Can you work these out from the drawing? Everything is in mm from the part's minimum corner. A direction names the side the tool comes from. Round coordinates to 2 decimals unless told otherwise and drop trailing zeros. Order: outer loops, then holes, each group sorted by start corner. A loop starts at its lowest first (then second) coordinate and runs counter-clockwise, first axis right, second up. Notation, with made-up numbers: (28, -23) - (56, -23) arc R28 cw to (56, 3) - close; hole circle Ø2 at (58.5, -0.75). An arc over 180 degrees is marked (long way). Write item = value, one per line.
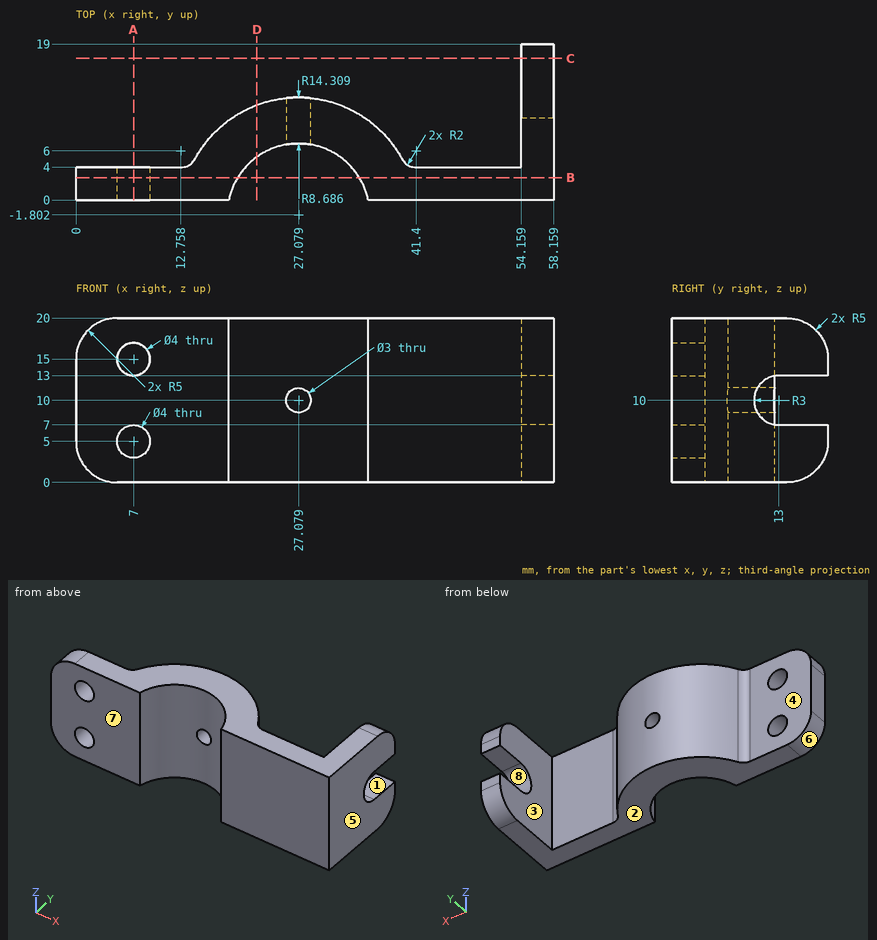
(1) On a 3-axis mill with a long thin cutter (end or side, diameter ignored), from which of +Z, -Z, +X, -X, +Y, -Y can I reach the whole of each face in a straight line? I mean the marked faces 1, 2, 3, 4 and 5. Say none if no direction works.
Computed:
face_1 = +X, -X, +Y
face_2 = -Z, +X, -X, +Y, -Y
face_3 = +Z, -Z, +Y
face_4 = +Z, -Z, -X, +Y
face_5 = +Z, -Z, +X, +Y, -Y
(2) Will these pins go through, and if not, where does the flat tip stop? P1, Ø3, axis at x = 56.5, y = 16, coming from the -Z side (1 decimal); P2, Ø10, axis at x = 6, z = 8, coming from the +Y side; P3, Ø3.5, axis at x = 7, z = 5, coming from the -Y side; P4, Ø5, axis at x = 7, z = 15, coming from the -Y side.
Computed:
P1 = 0
P2 = 4
P3 = through
P4 = 0
(3) If we section it at D-D (x = 22): Write out the boundary of the cut face in (y, z) (1 decimal).
Computed:
outline = (5.2, 0) - (11.6, 0) - (11.6, 20) - (5.2, 20) - close
(4) If we section it at B-B (y = 2.75): Write out the boundary of the cut face in (x, z).
Computed:
outline = (0, 5) arc R5 ccw to (5, 0) - (19.68, 0) - (19.68, 20) - (5, 20) arc R5 ccw to (0, 15) - close; (34.48, 0) - (58.16, 0) - (58.16, 20) - (34.48, 20) - close; hole circle Ø4 at (7, 5); hole circle Ø4 at (7, 15)
(5) If we section it at A-A (x = 7): Write out the boundary of the cut face in (y, z).
Computed:
outline = (0, 0) - (4, 0) - (4, 3) - (0, 3) - close; (0, 7) - (4, 7) - (4, 13) - (0, 13) - close; (0, 17) - (4, 17) - (4, 20) - (0, 20) - close
(6) Thinking about a two-plate mould opening in Z: for the marked faces 6, 7 and 8, which applies, +Z half, -Z half, draft (parallel to the pull), parting line (faces both ways), or undercut?
Computed:
face_6 = -Z half
face_7 = draft
face_8 = undercut
(7) If we section it at C-C (y = 17.25): Write out the boundary of the cut face in (x, z).
Computed:
outline = (54.16, 1.2) - (58.16, 1.2) - (58.16, 7) - (54.16, 7) - close; (54.16, 13) - (58.16, 13) - (58.16, 18.8) - (54.16, 18.8) - close
(8) If I drill on line 1 (Z direction, x = 7, y = 2.3); line 2 (X direction, y = 6, z = 14.75) (1 decimal); line 3 (X direction, y = 1.25, z = 15.75) (1 decimal), over which ranges is the centre line in solid material (lowest first)? Write a range as from..to.
Computed:
line_1 = 0..3, 7..13, 17..20
line_2 = 15.1..23.3, 30.9..39.1, 54.2..58.2
line_3 = 0.1..5.1, 8.9..18.9, 35.2..58.2
